The listing builds one solid part. Answer for the finished solid, in the listing's coordinates (mm). A direction names the side the tool comes from. Give positions to 0.01 mm unless a question says otherwise; leave off trailing zeros. Write each loop counter-clockwise with the first axis right and the second up, starting at its lowest first coordinate (ties: lowest second). Pieces come first, ordered by that corner, then holes. Notation, with made-up numbers: M 15.25,46.25 L 63.25,46.25 A27 cw 63.25,82.25 Z; hole C 85,-18 d4. An arc over 180 degrees is marked long. Answer as a JSON object with one key per item and string values.
```python
from build123d import *

# Parameters (mm, degrees)
F1_DEPTH = 12.7
F3_DEPTH = 12.7


with BuildPart() as f1:
    # F0 (on Front) → F1 (new body)
    with BuildSketch(Plane.XZ):
        Polygon((-132.122228, 16.423219), (-136.268499, 19.23676), (-141.444077, 19.888857), (-142.191744, 16.275135), (-140.710932, 10.20381), (-142.191744, 10.20381), (-142.191744, 7.53835), (-138.489716, 2.947835), (-136.416581, -1.050355), (-135.083851, -6.381276), (-133.751121, -11.712196), (-131.002761, -16.895032), (-125.606658, -21.342391), (-127.658351, -31.258902), (-131.002761, -33.523681), (-127.658351, -34.215628), (-127.658351, -35.276845), (-125.606658, -35.701333), (-123.977768, -35.701333), (-123.977768, -34.215628), (-116.128455, -34.215628), (-123.977768, -32.591632), (-122.200793, -24.002923), (-119.387253, -24.002923), (-114.500573, -22.374033), (-110.650467, -24.002923), (-105.763788, -32.591632), (-109.021573, -33.776282), (-105.763788, -33.776282), (-102.654087, -35.997501), (-102.654087, -33.776282), (-93.769217, -34.960932), (-93.769217, -33.776282), (-102.654087, -32.591632), (-107.985007, -24.002923), (-105.763788, -24.002923), (-102.654087, -20.597062), (-102.654087, -16.895032), (-97.471247, -14.081492), (-93.769217, -11.712196), (-90.067188, -6.381276), (-87.526385, 0.134294), (-85.624757, 5.613295), (-85.624757, 10.20381), (-87.526385, 13.511928), (-85.476677, 13.511928), (-83.717752, 16.71938), (-83.717752, 20.013939), (-81.490453, 18.792517), (-81.490453, 20.865652), (-81.490453, 25.634693), (-82.515056, 26.196572), (-82.515056, 28.875516), (-85.624757, 26.788895), (-85.624757, 31.866502), (-87.526385, 28.875516), (-90.067188, 30.490923), (-90.067188, 28.661053), (-91.103757, 28.875516), (-92.732648, 25.905185), (-91.103757, 25.011923), (-92.732648, 25.011923), (-96.882714, 22.295997), (-98.803977, 18.792517), (-101.321357, 14.202), (-104.282978, 10.648054), (-108.577332, 9.463405), (-112.575522, 10.648054), (-117.462198, 10.648054), (-121.164224, 10.648054), (-125.162414, 11.980785), (-129.456768, 14.202), align=None)
    extrude(amount=F1_DEPTH)

    # F2 (on face) → F3 (join)
    with BuildSketch(Plane.XZ.offset(12.7)):
        Polygon((-108.573183, -8.422106), (-108.573183, -4.432687), (-108.573183, -2.216344), (-119.211629, -2.216344), (-119.211629, -4.432687), (-119.211629, -8.422106), align=None)
    extrude(amount=F3_DEPTH)


solid = f1.part
```
1. A cutting plane is placed at A-A, the plane x = -123. Give the vertices of the cut face in (y, z), plus the area to 3 significant figures.
Verdict:
{"outline": "M -12.7,-34.22 L 0,-34.22 L 0,-32.79 L -12.7,-32.79 Z; M -12.7,-27.87 L 0,-27.87 L 0,11.26 L -12.7,11.26 Z", "area": "515 mm2"}
2. A cutting plane is placed at C-C, the plane y = -18.5. Give the vertices of the cut face in (x, z), plus the area to 3 significant figures.
Verdict:
{"outline": "M -119.21,-8.42 L -108.57,-8.42 L -108.57,-2.22 L -119.21,-2.22 Z", "area": "66.0 mm2"}
3. The mould has two halves that part along Z. Classify faces 1 (the flat face through (-95.646, -6.261, -12.913)), 2 (the flat face through (-112, -12.7, -2)), 3 (the flat face through (-129.354, -6.261, -33.865)): released by +Z, released by -Z, zero draft, split by the parting line, or undercut.
Verdict:
{"face 1": "undercut", "face 2": "zero draft", "face 3": "released by -Z"}
4. For faces 4 (the flat face through (-129.307, -6.261, -32.375)), 5 (the flat face through (-98.1, -6.3, -33.2)), 6 (the flat face through (-116.98, -6.26, -23.2)), 7 (the flat face through (-134.166, -6.261, 17.81)), 8 (the flat face through (-112.6, -6.26, -23.18)), determine the directions among +Z, -Z, +X, -X, +Y, -Y from which every point of the face is accessible in a straight line to the end or side of a thin tool.
Verdict:
{"face 4": "-X, +Y, -Y", "face 5": "+X, +Y, -Y", "face 6": "+Y, -Y", "face 7": "+Z, +Y, -Y", "face 8": "-Z, +Y, -Y"}
5. A cutting plane is placed at B-B, the plane z = -29. Give the vertices of the cut face in (x, y).
Verdict:
{"outline": "M -127.19,-12.7 L -123.23,-12.7 L -123.23,0 L -127.19,0 Z; M -107.81,-12.7 L -104.88,-12.7 L -104.88,0 L -107.81,0 Z"}
6. Consider line 1 along Z through (x, y) = (-107, -6.25); line 2 along Y through (x, z) = (-103, -9); line 3 along Z through (x, y) = (-121, -11.5). Determine where each line is inside the solid, lowest interval first.
Verdict:
{"line 1": "z = -33.78 to -33.04, -30.42 to -25.59, -24 to 9.9", "line 2": "y = -12.7 to 0", "line 3": "z = -34.22 to -33.21, -24 to 10.65"}
7. Flat-ended cylindrical pins translate along their axes: pin 1 (2.5 mm diameter, centred on y = -5.5, z = 29, fed in from +X); pin 2 (4 mm diameter, centred on x = -118.5, y = -8, fed in from -Z); pin 3 (1 mm diameter, centred on x = -107.5, y = -8.5, fed in from -Z). Find the tip coordinate at first contact, or state that the pin passes through.
Verdict:
{"pin 1": "stops at x = -82.52", "pin 2": "stops at z = -34.22", "pin 3": "stops at z = -33.78"}
8. A cutting plane is placed at D-D, the plane z = -4. Give the vertices of the cut face in (x, y), plus the area to 3 significant figures.
Verdict:
{"outline": "M -135.68,-12.7 L -119.21,-12.7 L -119.21,-25.4 L -108.57,-25.4 L -108.57,-12.7 L -89.14,-12.7 L -89.14,0 L -135.68,0 Z", "area": "726 mm2"}
